from build123d import *

# Parameters (mm, degrees)
F1_DEPTH = 225
F3_DEPTH = 25


with BuildPart() as f1:
    # F0 (on Right) → F1 (new body)
    with BuildSketch(Plane.YZ):
        Polygon((150, 220), (150, 250), (0, 250), (0, 220), (10, 220), (10, 240), (140, 240), (140, 220), align=None)
    extrude(amount=F1_DEPTH)



with BuildPart() as f1b:
    # F0 (on Right) → F1, piece 2 (new body)
    with BuildSketch(Plane.YZ):
        Polygon((160, 470), (160, 490), (290, 490), (290, 470), (300, 470), (300, 500), (150, 500), (150, 470), align=None)
    extrude(amount=F1_DEPTH)


with BuildPart() as f1c:
    # F0 (on Right) → F1, piece 3 (new body)
    with BuildSketch(Plane.YZ):
        Polygon((300, 750), (300, 720), (310, 720), (310, 740), (590, 740), (590, 720), (600, 720), (600, 750), align=None)
    extrude(amount=F1_DEPTH)


with BuildPart() as f1_1:
    add(f1.part)

    add(f1b.part)  # F3 merges F1b

    add(f1c.part)  # F3 merges F1c
    # F2 (on face) → F3 (join)
    with BuildSketch(Plane.YZ.offset(225)):
        Polygon((600, 0), (600, 750), (345.8452405258, 750), (-104.1547594742, 0), (-45.8452405258, 0), (374.1547594742, 700), (550, 700), (550, 0), align=None)
    extrude(amount=F3_DEPTH)

    # F4: F1 across plane


with BuildPart() as f1_2:
    add(f1_1.part)
    add(f1_1.part.mirror(Plane.YZ))


solid = f1_2.part
Can you work these out from the model? Positions are in its coordinate system, mm. A direction names the side the tool comes from. Give positions to 0.01 mm unless a question says otherwise; leave off trailing zeros. Order: outer loops, then holes, each group sorted by start corner. A loop starts at its lowest first (then second) coordinate and runs counter-clockwise, first axis right, second up. Notation, with made-up numbers: M -14.75,85 L 6.25,85 A17 cw 6.25,98 Z; hole C -31.5,1.5 d9. An arc over 180 degrees is marked long. Use a Markdown table: item, result. Add a question column.
Item 1: If I drill on L1, parallel to X at y = 262, z = 598; L2, parallel to Y at x = -153.5, z = 229; L3, parallel to Z at x = -136, y = 270, over which ranges is the centre line in solid material (lowest first)? Write a range as [from, to].
Item 2: Suppose I cut it at B-B (z = 137). List the corners of the cut face in (x, y) for me, then the cut area to 3 significant figures.
Item 3: We'd pull the mould along X, two halves only. Please class faces 6 (the flat face through (-225, 18, 242)), 7 (the flat face through (-240, 600, 484)), 8 (the flat face through (225, 18, 242)), 9 (the flat face through (3, 74, 240)): +X half, -X half, draft (parallel to the pull), parting line (faces both ways), or undercut.
Item 4: Suppose I cut it at A-A (x = 110). List the corners of the cut face in (y, z) for me, then the cut area to 3 significant figures.
Item 5: Will these pins go through, and if not, where does the flat tip stop? pin 1 (2 mm diameter, centred on x = -177, y = 145, fed in from -Z); pin 2 (10 mm diameter, centred on x = -100, z = 727, fed in from -Y); pin 3 (6 mm diameter, centred on x = -170.5, y = 424, fed in from -Z).
Item 6: For faces 1 (the flat face through (3, 76, 250)), 2 (the flat face through (225, 168, 492)), 3 (the flat face through (225, 279, 492)), 4 (the flat face through (3, 150, 485)), 5 (the flat face through (237, 461, 700)), which set-ups out of +Z, -Z, +X, -X, +Y, -Y let a thin tool reach every point of the face, with its end or its side?
Answer sheet:
| question | item | result |
|---|---|---|
| 1 | L1 | x = [-250, -225], [225, 250] |
| 1 | L2 | y = [0, 10], [140, 150] |
| 1 | L3 | z = [490, 500] |
| 2 | outline | M -250,-21.95 L -225,-21.95 L -225,36.35 L -250,36.35 Z; M -250,550 L -225,550 L -225,600 L -250,600 Z; M 225,-21.95 L 250,-21.95 L 250,36.35 L 225,36.35 Z; M 225,550 L 250,550 L 250,600 L 225,600 Z |
| 2 | area | 5,420 mm² |
| 3 | face 6 | -X half |
| 3 | face 7 | draft |
| 3 | face 8 | +X half |
| 3 | face 9 | undercut |
| 4 | outline | M 0,220 L 10,220 L 10,240 L 140,240 L 140,220 L 150,220 L 150,250 L 0,250 Z; M 150,470 L 160,470 L 160,490 L 290,490 L 290,470 L 300,470 L 300,500 L 150,500 Z; M 300,720 L 310,720 L 310,740 L 590,740 L 590,720 L 600,720 L 600,750 L 300,750 Z |
| 4 | area | 7,200 mm² |
| 5 | pin 1 | stops at z = 220 |
| 5 | pin 2 | stops at y = 300 |
| 5 | pin 3 | stops at z = 740 |
| 6 | face 1 | +Z, +Y, -Y |
| 6 | face 2 | +Z, +X, -Y |
| 6 | face 3 | -Z, +X |
| 6 | face 4 | +Z, +X, -X, -Y |
| 6 | face 5 | -Z, +X, -X |
